```python
from build123d import *

# Parameters (mm, degrees)
F0_W      = 50
F0_H      = 20
F1_DEPTH  = 20
F4_DEPTH  = 50
F5_W      = 10
F5_H      = 10
F6_DEPTH  = 5
F7_W      = 10
F7_H      = 5
F8_DEPTH  = 10
F9_W      = 10
F9_H      = 5
F10_DEPTH = 50
F12_W     = 10
F12_H     = 5
F13_DEPTH = 10
F14_W     = 10
F14_H     = 10
F15_DEPTH = 5
F16_W     = 10
F16_H     = 10
F17_DEPTH = 5


with BuildPart() as f1:
    # F0 (on Right) → F1 (new body)
    with BuildSketch(Plane.YZ):
        with Locations((25, -10)):
            Rectangle(F0_W, F0_H)
    extrude(amount=F1_DEPTH)

    # F3 (on offset) → F4 (join)
    with BuildSketch(Plane(origin=(0, 50, 0), x_dir=(-1, 0, 0), z_dir=(0, 1, 0))):
        with BuildLine():
            ThreePointArc((31.9188415439, -32.6248712805), (35.1568284949, -34.0445333899), (36.5764906043, -30.8065464388))
            ThreePointArc((36.5764906043, -30.8065464388), (-10, 1.0102051443), (-56.5764906043, -30.8065464388))
            ThreePointArc((-56.5764906043, -30.8065464388), (-55.1568284949, -34.0445333899), (-51.9188415439, -32.6248712805))
            ThreePointArc((-51.9188415439, -32.6248712805), (-10, -3.9897948557), (31.9188415439, -32.6248712805))
        make_face()
    extrude(amount=-F4_DEPTH)

    # F5 (on offset) → F6 (cut)
    with BuildSketch(Plane(origin=(0, 50, 0), x_dir=(-1, 0, 0), z_dir=(0, 1, 0))):
        with Locations((-10, -10)):
            Rectangle(F5_W, F5_H)
    extrude(amount=-F6_DEPTH, mode=Mode.SUBTRACT)

    # F7 (on offset) → F8 (cut)
    with BuildSketch(Plane(origin=(0, 50, 0), x_dir=(-1, 0, 0), z_dir=(0, 1, 0))):
        with Locations((-10, -7.5)):
            Rectangle(F7_W, F7_H)
    extrude(amount=-F8_DEPTH, mode=Mode.SUBTRACT)

    # F9 (on offset) → F10 (cut)
    with BuildSketch(Plane(origin=(0, 50, 0), x_dir=(-1, 0, 0), z_dir=(0, 1, 0))):
        with Locations((-10, -17.5)):
            Rectangle(F9_W, F9_H)
    extrude(amount=-F10_DEPTH, mode=Mode.SUBTRACT)

    # F12 (on offset) → F13 (cut)
    with BuildSketch(Plane(origin=(0, 20, 0), x_dir=(-1, 0, 0), z_dir=(0, 1, 0))):
        with Locations((-10, -7.5)):
            Rectangle(F12_W, F12_H)
    extrude(amount=-F13_DEPTH, mode=Mode.SUBTRACT)

    # F14 (on offset) → F15 (cut)
    with BuildSketch(Plane(origin=(0, 20, 0), x_dir=(-1, 0, 0), z_dir=(0, 1, 0))):
        with Locations((-10, -10)):
            Rectangle(F14_W, F14_H)
    extrude(amount=-F15_DEPTH, mode=Mode.SUBTRACT)

    # F16 (on offset) → F17 (cut)
    with BuildSketch(Plane(origin=(0, 20, 0), x_dir=(-1, 0, 0), z_dir=(0, 1, 0))):
        with Locations((-10, -10)):
            Rectangle(F16_W, F16_H)
    extrude(amount=F17_DEPTH, mode=Mode.SUBTRACT)


solid = f1.part
```
Model file for the job. Use its own axes, mm. A direction names the side the tool comes from. Coordinates: 2 decimals unless noted, no trailing zeros. Order: outer loops, then holes, each group sorted by start corner. A loop starts at its lowest first (then second) coordinate and runs counter-clockwise, first axis right, second up. Notation, with made-up numbers: M -40,16 L -4,16 A6 ccw -4,24 Z; hole C 62,8 d6. An arc over 180 degrees is marked long. Answer as CSV lines item,"result".
(1) Band-saw the part on B-B, the plane z = -29. List the corners of the cut face in (x, y).
Geometry says:
outline,"M -35.83,0 L -30.32,0 L -30.32,50 L -35.83,50 Z; M 50.32,0 L 55.83,0 L 55.83,50 L 50.32,50 Z"
(2) Band-saw the part on D-D, the plane y = 27.5. List the corners of the cut face in (x, z), then the cut area to 3 significant figures.
Geometry says:
outline,"M -36.58,-30.81 A2.5 ccw -31.92,-32.62 A45 cw 0,-5.11 L 0,-20 L 5,-20 L 5,-15 L 15,-15 L 15,-20 L 20,-20 L 20,-5.11 A45 cw 51.92,-32.62 A2.5 ccw 56.58,-30.81 A50 ccw Z"
area,"852 mm2"
(3) Band-saw the part on C-C, the plane x = 8. List the corners of the cut face in (y, z).
Geometry says:
outline,"M 0,-15 L 15,-15 L 15,-10 L 10,-10 L 10,-5 L 25,-5 L 25,-15 L 45,-15 L 45,-10 L 40,-10 L 40,-5 L 50,-5 L 50,0.97 L 0,0.97 Z"
(4) Flat gauge pins, fed straight in: pin 1 (4 mm diameter, centred on x = 27, y = 7, fed in from -Z); pin 2 (3 mm diameter, centred on x = 9.5, y = 32, fed in from -Z); pin 3 (4.5 mm diameter, centred on y = 16, z = -14.5, fed in from -X). Where does each tip first touch, or does it go through?
Geometry says:
pin 1,"stops at z = -8.2"
pin 2,"stops at z = -15"
pin 3,"stops at x = -28.22"
(5) Band-saw the part on A-A, the plane y = 12.5. List the corners of the cut face in (x, z).
Geometry says:
outline,"M -36.58,-30.81 A2.5 ccw -31.92,-32.62 A45 cw 0,-5.11 L 0,-20 L 5,-20 L 5,-15 L 15,-15 L 15,-20 L 20,-20 L 20,-5.11 A45 cw 51.92,-32.62 A2.5 ccw 56.58,-30.81 A50 ccw Z; hole M 5,-10 L 15,-10 L 15,-5 L 5,-5 Z"
(6) Wall check: line 1 along X through (y, z) = (19, -17.5); line 2 along X through (y, z) = (32, -8.5); line 3 along X through (y, z) = (7, -9.5). Give the ranges that are in metal, low to high.
Geometry says:
line 1,"x = -28.84 to -22.15, 0 to 5, 15 to 20, 42.15 to 48.84"
line 2,"x = -19.34 to -9.64, 0 to 20, 29.64 to 39.34"
line 3,"x = -20.67 to -11.58, 0 to 20, 31.58 to 40.67"
(7) 3-axis set-ups, long thin cutter, end or side, ignore diameter. For faces 1 (the flat face through (10, 45, -5)), 2 (the flat face through (10, 15, -12)), 3 (the flat face through (0, 25, -12)): which of +Z, -Z, +X, -X, +Y, -Y reach the whole face in a straight line?
Geometry says:
face 1,"+Y"
face 2,"-Z"
face 3,"-Z, +Y, -Y"
(8) Pull direction Y, two halves, no side cores. Call faces 4 (the flat face through (10, 25, -10)), 5 (the flat face through (5, 25, -16)), 6 (the flat face through (10, 35, -15)), 7 (the flat face through (10, 45, -12)): +Y half, -Y half, draft (parallel to the pull), parting line (faces both ways), or undercut.
Geometry says:
face 4,"undercut"
face 5,"undercut"
face 6,"draft"
face 7,"+Y half"
